Verification items for the finished model (mm, model axes). Face numbers are marked on the shaded views. A direction names the side the tool comes from. Coordinates: 2 decimals unless noted, no trailing zeros. Order: outer loops, then holes, each group sorted by start corner. A loop starts at its lowest first (then second) coordinate and runs counter-clockwise, first axis right, second up. Notation, with made-up numbers: M -10.75,-4.75 L 35.25,-4.75 A21 ccw 35.25,28.25 Z; hole C 5.5,46 d8. An arc over 180 degrees is marked long. Return JSON: item names as keys, results as strings. Group by question number.
1. Material ranges on line 1 along X through (y, z) = (1.05, 0); line 2 along Z through (x, y) = (17.78, 2.35) (3 decimals); line 3 along Y through (x, z) = (-1.5, 0) (3 decimals), recorded low to high.
2. Set-up check for the marked faces 1, 2 and 3: record each of +Z, -Z, +X, -X, +Y, -Y from which the full face is reachable in a straight line by a thin tool's end or side.
3. Section check A-A, the plane z = 0. Record the cut outline in (x, y) (3 decimals).
4. Section check C-C, the plane y = 2.5. Record the cut outline in (x, z) (3 decimals), plus the area to 3 significant figures.
5. Section check D-D, the plane z = -4.5. Record the cut outline in (x, y) (3 decimals), plus the area to 3 significant figures.
6. Gauge pin test, flat ends, axial feed: pin 1 (6 mm diameter, centred on x = -17, z = 7, fed in from +Y) (3 decimals); pin 2 (3 mm diameter, centred on y = 23, z = -2.5, fed in from +X). Record the tip position at first contact, or that the pin passes through.
7. Mould release check, pull along X, two halves, no side actions. Record for the marked faces 4, 5 and 6: +X half, -X half, draft (parallel to the pull), parting line (faces both ways), or undercut.
8. Section check B-B, the plane x = 17.78. Record the cut outline in (y, z) (3 decimals).
```python
from build123d import *

# Parameters (mm, degrees)
SKETCH1_W               = 50.8
SKETCH1_H               = 19.05
BOSS_EXTRUDE1_DEPTH     = 3.175
SKETCH2_W               = 7.874
SKETCH2_H               = 19.05
BOSS_EXTRUDE2_DEPTH     = 30.48
CUT_EXTRUDE1_DEPTH      = 46.651333157
CUT_EXTRUDE1_DEPTH_BACK = 46.651333157
SKETCH3_R               = 3.937
CUT_EXTRUDE2_DEPTH      = 41.803382519
CUT_EXTRUDE2_DEPTH_BACK = 41.803382519
SKETCH5_R               = 3.302
FILLET2_R               = 2.54


with BuildPart() as part:
    # Sketch1 → Boss-Extrude1 (new body)
    with BuildSketch(Plane(origin=(0, 0, 0), x_dir=(1, 0, 0), z_dir=(0, 1, 0))):
        Rectangle(SKETCH1_W, SKETCH1_H)
    extrude(amount=BOSS_EXTRUDE1_DEPTH)

    # Sketch2 → Boss-Extrude2 (add)
    with BuildSketch(Plane(origin=(0, 3.175, 0), x_dir=(1, 0, 0), z_dir=(0, 1, 0))):
        Rectangle(SKETCH2_W, SKETCH2_H)
    extrude(amount=BOSS_EXTRUDE2_DEPTH)

    # Sketch3 → Cut-Extrude1 (cut, two sides: drawn at the far end of the back side and taken through both)
    with BuildSketch(Plane(origin=(3.937, 0, 0), x_dir=(0, 0, -1), z_dir=(1, 0, 0)).offset(-CUT_EXTRUDE1_DEPTH_BACK)):
        with Locations((0, 23.495)):
            Circle(SKETCH3_R)
    extrude(amount=CUT_EXTRUDE1_DEPTH + CUT_EXTRUDE1_DEPTH_BACK, mode=Mode.SUBTRACT)

    # Sketch5 → Cut-Extrude2 (cut, two sides: drawn at the far end of the back side and taken through both)
    with BuildSketch(Plane(origin=(0, 3.175, 0), x_dir=(1, 0, 0), z_dir=(0, 1, 0)).offset(-CUT_EXTRUDE2_DEPTH_BACK)):
        with Locations(Location((-17.78, 0, 0), (0, 0, 270))):
            Circle(SKETCH5_R)
        with Locations(Location((17.78, 0, 0), (0, 0, 270))):
            Circle(SKETCH5_R)
    extrude(amount=CUT_EXTRUDE2_DEPTH + CUT_EXTRUDE2_DEPTH_BACK, mode=Mode.SUBTRACT)

    # Fillet2
    fillet2_edges = [part.edges().sort_by_distance(p)[0] for p in [
        (0, 33.655, -9.525),
        (0, 33.655, 9.525),
        (25.4, 1.5875, 9.525),
        (-25.4, 1.5875, 9.525),
        (-25.4, 1.5875, -9.525),
        (25.4, 1.5875, -9.525),
    ]]
    fillet(fillet2_edges, radius=FILLET2_R)


solid = part.part
```
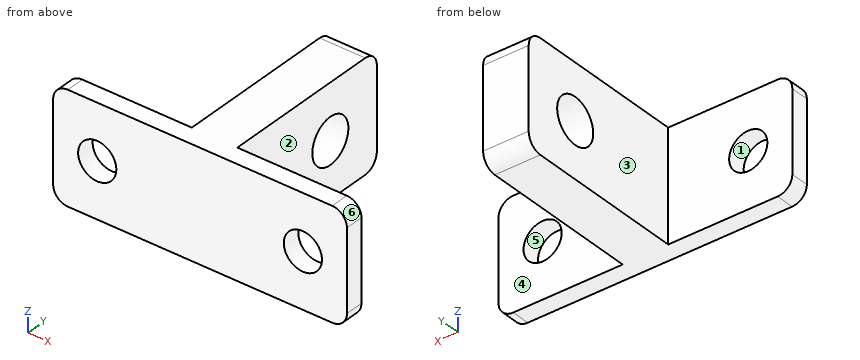
Answers follow:
{
 "1": {"line 1": "-25.4 to -21.08, -14.48 to 14.48, 21.08 to 25.4", "line 2": "-9.525 to -3.302, 3.302 to 9.525", "line 3": "0 to 19.558, 27.432 to 33.655"},
 "2": {"face 1": "+Y, -Y", "face 2": "+Z, -Z, +X, +Y", "face 3": "+Z, -Z, -X, +Y"},
 "3": {"outline": "M -25.4,0 L -21.082,0 L -21.082,3.175 L -25.4,3.175 Z; M -14.478,0 L 14.478,0 L 14.478,3.175 L 3.937,3.175 L 3.937,19.558 L -3.937,19.558 L -3.937,3.175 L -14.478,3.175 Z; M -3.937,27.432 L 3.937,27.432 L 3.937,33.655 L -3.937,33.655 Z; M 21.082,0 L 25.4,0 L 25.4,3.175 L 21.082,3.175 Z"},
 "4": {"outline": "M -25.4,-6.985 A2.54 ccw -22.86,-9.525 L 22.86,-9.525 A2.54 ccw 25.4,-6.985 L 25.4,6.985 A2.54 ccw 22.86,9.525 L -22.86,9.525 A2.54 ccw -25.4,6.985 Z; hole C -17.78,0 d6.604; hole C 17.78,0 d6.604", "area": "894 mm^2"},
 "5": {"outline": "M -25.4,0 L 25.4,0 L 25.4,3.175 L 3.937,3.175 L 3.937,33.655 L -3.937,33.655 L -3.937,3.175 L -25.4,3.175 Z", "area": "401 mm^2"},
 "6": {"pin 1": "y = 3.175", "pin 2": "x = 3.94"},
 "7": {"face 4": "draft", "face 5": "undercut", "face 6": "+X half"},
 "8": {"outline": "M 0,-9.525 L 3.175,-9.525 L 3.175,-3.302 L 0,-3.302 Z; M 0,3.302 L 3.175,3.302 L 3.175,9.525 L 0,9.525 Z"}
}
